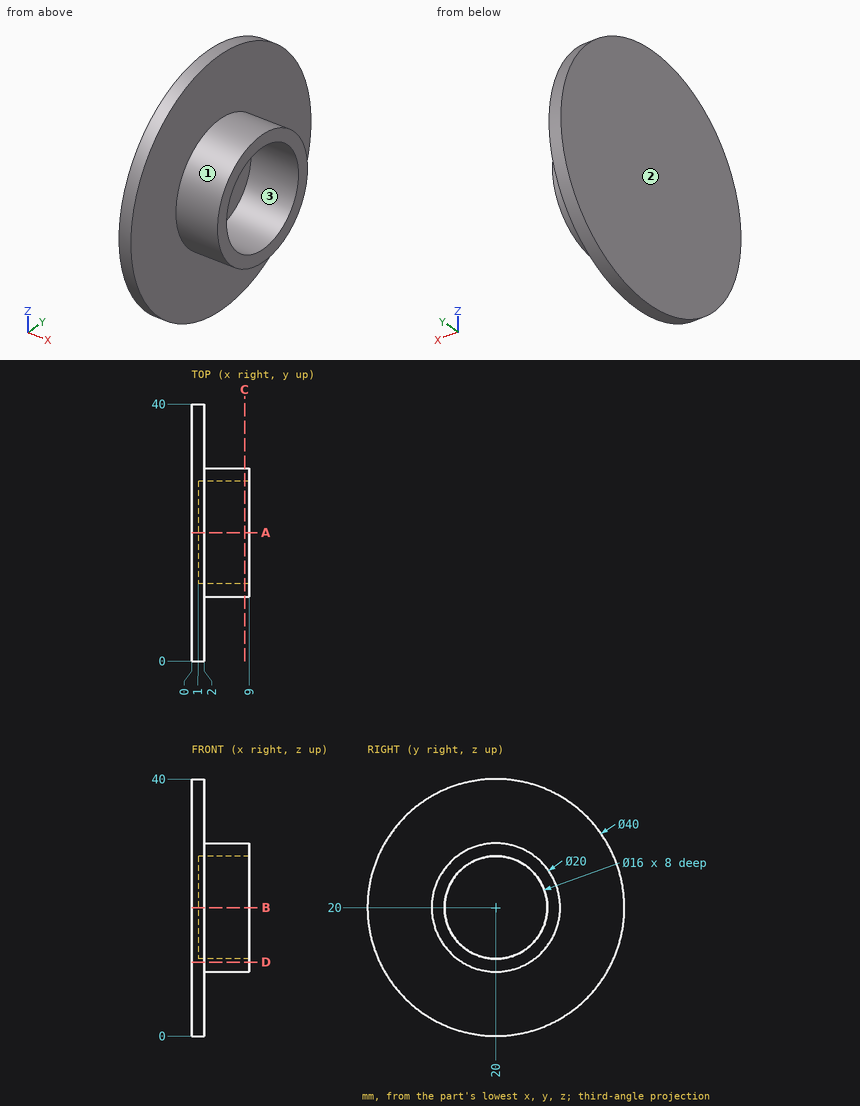
Input: dimensioned drawing with shaded views. Units: mm. Origin: part minimum x, y, z. Coordinates: 2 decimals unless noted, no trailing zeros. Order: outer loops, then holes, each group sorted by start corner. A loop starts at its lowest first (then second) coordinate and runs counter-clockwise, first axis right, second up. Notation, with made-up numbers: M 21.25,52.5 L 79.25,52.5 A20 cw 79.25,77.5 Z; hole C 15,35.25 d3. An arc over 180 degrees is marked long. Write each question's results on one line, items separated by ' | '. Start each with the question number.
Item 1: Cut plane A-A (y = 20). Return loops of the section in (x, z).
Item 2: Cut plane D-D (z = 11.5). Return loops of the section in (x, y), and give its area (3 significant figures).
Item 3: First-contact query: pin 1 Ø8 at (y, z) = (7, 31) entering from +X; pin 2 Ø2 at (x, y) = (4, 23) entering from +Z. Flat tips, straight axial feed; report the tip coordinate or a pass-through.
Item 4: Draft query along Z for the marked faces 1, 2 and 3. Return one class per face: pulls with the +Z half, pulls with the -Z half, needs draft (parallel to the pull), parting line crosses it, or undercut.
Item 5: Line query: probe 1 along Y at (x, z) = (4.25, 20); probe 2 along X at (y, z) = (25.5, 4). Output: solid intervals per line, ascending.
Item 6: Cut plane C-C (x = 8.25). Return loops of the section in (y, z), and give its area (3 significant figures).
Checked values:
1) outline: M 0,0 L 2,0 L 2,10 L 9,10 L 9,12 L 1,12 L 1,28 L 9,28 L 9,30 L 2,30 L 2,40 L 0,40 Z
2) outline: M 0,1.9 L 2,1.9 L 2,14.73 L 9,14.73 L 9,25.27 L 2,25.27 L 2,38.1 L 0,38.1 Z | area: 146 mm2
3) pin 1: stops at x = 2 | pin 2: stops at z = 29.8
4) face 1: parting line crosses it | face 2: needs draft | face 3: undercut
5) probe 1: y = 10 to 12, 28 to 30 | probe 2: x = 0 to 2
6) outline: C 20,20 d20; hole C 20,20 d16 | area: 113 mm2
